from build123d import *

# Parameters (mm, degrees)
F0_W    = 13.5
F0_H    = 15
F2_SIZE = 0.635


with BuildPart() as f1:
    # F0 (on Front) → F1 (revolve)
    with BuildSketch(Plane.XZ):
        with Locations((-19.25, 0)):
            Rectangle(F0_W, F0_H)
    revolve(axis=Axis((0, 0, 3.400517), (0, 0, -1)))

    # F2
    f2_edges = [f1.edges().sort_by_distance(p)[0] for p in [
        (26, 0, 7.5),
        (26, 0, -7.5),
        (12.5, 0, 7.5),
        (12.5, 0, -7.5),
    ]]
    chamfer(f2_edges, length=F2_SIZE)


solid = f1.part
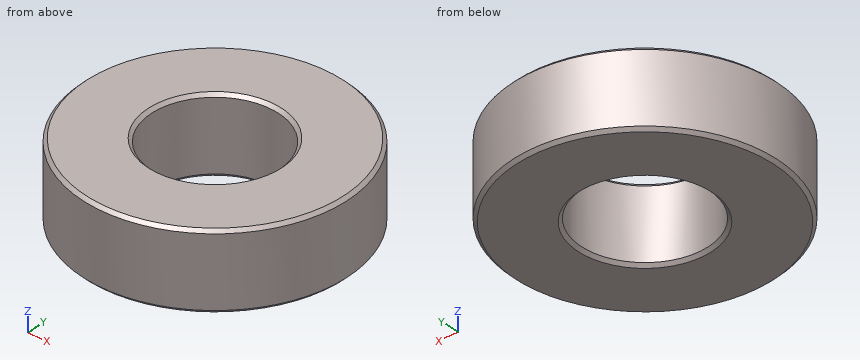
Read the model definition and answer for the solid it produces. Units are mm, in the model's axes. Give positions to 0.01 mm unless a question says otherwise; leave off trailing zeros. Loops run counter-clockwise (first coordinate to the right, second up) from the corner with the lowest first, then second, coordinate; pieces in that order, holes last. Notation, with made-up numbers: (-24.75, 54) - (32.25, 54) arc R23 ccw to (32.25, 87) - close; hole circle Ø5 at (49.25, 36). An arc over 180 degrees is marked (long way). Answer as CSV lines item,"result". Start each with the question number.
1) Each of these flat-tipped pins is pushed along its axis until it touches: pin 1 Ø3 at (x, y) = (-16.5, 20.5) entering from -Z; pin 2 Ø1.5 at (y, z) = (13.5, -2) entering from +X; pin 3 Ø1.5 at (y, z) = (-6, 2.5) entering from -X; pin 4 Ø5 at (x, z) = (-8, 4.5) entering from +Y. Where does it stop, or does it pass through?
2) Find section A-A (x = 0). Write down the section's boundary in (y, z) (3 decimals).
3) Straight lines are drawn through the part: L1, parallel to Y at x = 0, z = 0.5; L2, parallel to Y at x = -8.5, z = -5; L3, parallel to X at y = 1, z = -4.5. For each, find the intervals that lie inside material, in ascending order. Write a range as from..to.
4) Find section C-C (z = -2.5). Write down the section's boundary in (x, y), then the cut area to 3 significant figures.
Findings below:
1,pin 1,"z = -7.5"
1,pin 2,"x = 22.66"
1,pin 3,"x = -25.46"
1,pin 4,"y = 25.41"
2,outline,"(-26, -6.865) - (-25.365, -7.5) - (-13.135, -7.5) - (-12.5, -6.865) - (-12.5, 6.865) - (-13.135, 7.5) - (-25.365, 7.5) - (-26, 6.865) - close; (12.5, -6.865) - (13.135, -7.5) - (25.365, -7.5) - (26, -6.865) - (26, 6.865) - (25.365, 7.5) - (13.135, 7.5) - (12.5, 6.865) - close"
3,L1,"-26..-12.5, 12.5..26"
3,L2,"-24.57..-9.17, 9.17..24.57"
3,L3,"-25.98..-12.46, 12.46..25.98"
4,outline,"circle Ø52 at (0, 0); hole circle Ø25 at (0, 0)"
4,area,"1,630 mm^2"
